Design review of the part built by this model. Coordinates are the model's own, in mm. Face numbers are marked on the shaded views. A direction names the side the tool comes from. Give positions to 0.01 mm unless a question says otherwise; leave off trailing zeros. Loops run counter-clockwise (first coordinate to the right, second up) from the corner with the lowest first, then second, coordinate; pieces in that order, holes last. Notation, with made-up numbers: (87, -15) -> (146, -15) arc R22 cw to (146, 6) -> close; hole circle Ø7 at (49, 56). An arc over 180 degrees is marked (long way). Use a Markdown table: item, result. Add a question column.
1. Draft analysis for pull direction Y (two halves, no side actions). For the marked faces 1, 2, 3 and 4, state which applies: pulls with the +Y half, pulls with the -Y half, needs draft (parallel to the pull), parting line crosses it, or undercut.
2. Add section A-A (z = 0). State the section outline as (x, y) points.
3. For pin 1 Ø1 at (x, y) = (32, 17) entering from +Z; pin 2 Ø10 at (x, y) = (28, 5.5) entering from +Z; pin 3 Ø6 at (y, z) = (10.5, -27) entering from +X; pin 4 Ø3 at (x, z) = (33.5, -3.5) entering from -Y, all flat-tipped, find the tip position at first contact; note any pin that passes through.
4. To check wall thickness, follow line 1 (Z direction, x = 22, y = 8); line 2 (Z direction, x = 22, y = 17); line 3 (X direction, y = 19.5, z = 0). State the ranges of each line that lie inside material, in increasing order.
5. For the marked faces 5 and 6, list the 3-axis set-ups (+Z, -Z, +X, -X, +Y, -Y) from which the entire face can be reached by the end or side of a thin tool; tool diameter is ignored.
6. Add section B-B (x = 22.5). State the section outline as (y, z) points, and give its area (3 significant figures).
7. Add section C-C (y = 12.5). State the section outline as (x, z) points.
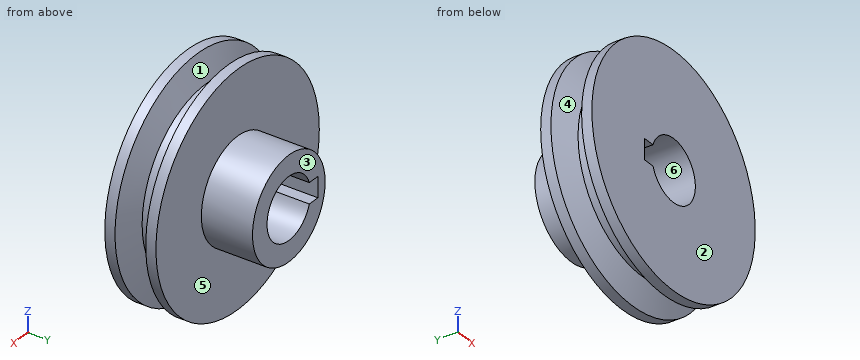
```python
from build123d import *

# Parameters (mm, degrees)
SKETCH2_R          = 12
CUT_EXTRUDE1_DEPTH = 91.450262576
SKETCH3_W          = 16
SKETCH3_H          = 8
CUT_EXTRUDE2_DEPTH = 91.450262576


with BuildPart() as part:
    # Sketch1 → Revolve1 (revolve)
    with BuildSketch(Plane.XY):
        Polygon((-12.5, 2.5), (-12.5, -2.5), (-22.5, -6), (-22.5, -10), (22.5, -10), (22.5, 10), (22.5, 30), (2.5, 30), (2.5, 10), (-22.5, 10), (-22.5, 6), align=None)
    revolve(axis=Axis((22.5, 43.956272641, 0), (0, -1, 0)))

    # Sketch2 → Cut-Extrude1 (cut, through all)
    with BuildSketch(Plane(origin=(0, 30, 0), x_dir=(1, 0, 0), z_dir=(0, 1, 0))):
        with Locations(Location((22.5, 0, 0), (0, 0, 180))):
            Circle(SKETCH2_R)
    extrude(amount=-CUT_EXTRUDE1_DEPTH, mode=Mode.SUBTRACT)

    # Sketch3 → Cut-Extrude2 (cut, through all)
    with BuildSketch(Plane(origin=(0, 30, 0), x_dir=(1, 0, 0), z_dir=(0, 1, 0))):
        with Locations((14.5, 0)):
            Rectangle(SKETCH3_W, SKETCH3_H)
    extrude(amount=-CUT_EXTRUDE2_DEPTH, mode=Mode.SUBTRACT)


solid = part.part
```
Taken from the geometry:
| question | item | result |
|---|---|---|
| 1 | face 1 | undercut |
| 1 | face 2 | pulls with the -Y half |
| 1 | face 3 | pulls with the +Y half |
| 1 | face 4 | undercut |
| 2 | outline | (-22.5, -10) -> (6.5, -10) -> (6.5, 30) -> (2.5, 30) -> (2.5, 10) -> (-22.5, 10) -> (-22.5, 6) -> (-12.5, 2.5) -> (-12.5, -2.5) -> (-22.5, -6) -> close; (34.5, -10) -> (67.5, -10) -> (67.5, -6) -> (57.5, -2.5) -> (57.5, 2.5) -> (67.5, 6) -> (67.5, 10) -> (42.5, 10) -> (42.5, 30) -> (34.5, 30) -> close |
| 3 | pin 1 | stops at z = 17.86 |
| 3 | pin 2 | stops at z = 45 |
| 3 | pin 3 | stops at x = 60.54 |
| 3 | pin 4 | stops at y = -10 |
| 4 | line 1 | z = -45 to -11.99, 11.99 to 45 |
| 4 | line 2 | z = -19.99 to -11.99, 11.99 to 19.99 |
| 4 | line 3 | x = 2.5 to 6.5, 34.5 to 42.5 |
| 5 | face 5 | +Y |
| 5 | face 6 | +Y, -Y |
| 6 | outline | (-10, -45) -> (-6, -45) -> (-2.5, -35) -> (2.5, -35) -> (6, -45) -> (10, -45) -> (10, -20) -> (30, -20) -> (30, -12) -> (-10, -12) -> close; (-10, 12) -> (30, 12) -> (30, 20) -> (10, 20) -> (10, 45) -> (6, 45) -> (2.5, 35) -> (-2.5, 35) -> (-6, 45) -> (-10, 45) -> close |
| 6 | area | 1,470 mm^2 |
| 7 | outline | circle Ø40 at (22.5, 0); hole (6.5, -4) -> (11.19, -4) arc R12 ccw (long way) to (11.19, 4) -> (6.5, 4) -> close |
